The drawing under review shows one solid part. Ordinate dimensions are in mm from its lowest x, y, z. A direction names the side the tool comes from. Give positions to 0.01 mm unless a question says otherwise; leave off trailing zeros. Order: outer loops, then holes, each group sorted by start corner. A loop starts at its lowest first (then second) coordinate and runs counter-clockwise, first axis right, second up. Notation, with made-up numbers: (-14.75, -12) - (37.25, -12) arc R23 ccw to (37.25, 12) - close; hole circle Ø2 at (2.5, -20.5). An arc over 180 degrees is marked (long way). Use CSV: the item, a comma, the result in double quotes.
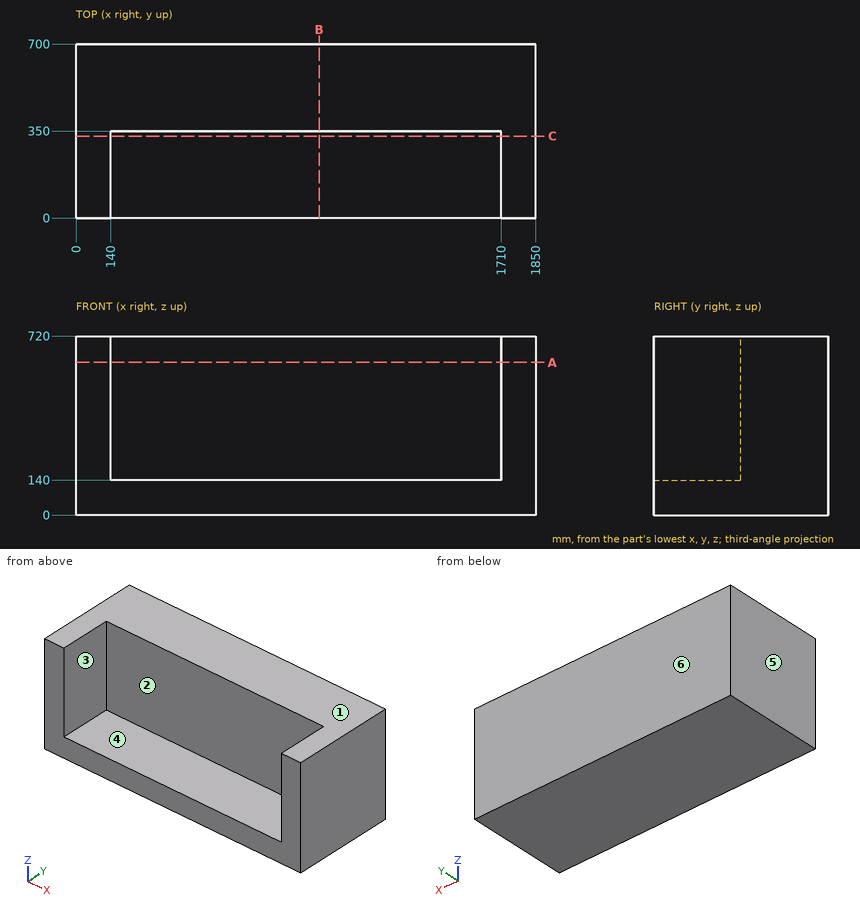
Item 1: Take a section at B-B, the plane x = 977.5. Give the boundary of the cut face in (y, z), and give its area (3 significant figures).
Results list:
outline,"(0, 0) - (700, 0) - (700, 720) - (350, 720) - (350, 140) - (0, 140) - close"
area,"301,000 mm2"
Item 2: Clearance check with a flat-ended pin moving along its axis: pin 1 (10 mm diameter, centred on x = 465, y = 264.5, fed in from +Z). State where the tip first meets the part, or that it passes through.
Results list:
pin 1,"stops at z = 140"
Item 3: Take a section at C-C, the plane y = 329.5. Give the boundary of the cut face in (x, z), and give its area (3 significant figures).
Results list:
outline,"(0, 0) - (1850, 0) - (1850, 720) - (1710, 720) - (1710, 140) - (140, 140) - (140, 720) - (0, 720) - close"
area,"421,000 mm2"
Item 4: Take a section at A-A, the plane z = 614.5. Give the boundary of the cut face in (x, y).
Results list:
outline,"(0, 0) - (140, 0) - (140, 350) - (1710, 350) - (1710, 0) - (1850, 0) - (1850, 700) - (0, 700) - close"
Item 5: Tool access review of the marked faces 1 and 2: name each direction out of +Z, -Z, +X, -X, +Y, -Y from which nothing blocks a thin tool from reaching the whole face with its end or side.
Results list:
face 1,"+Z, +X, -X, +Y, -Y"
face 2,"+Z, -Y"
Item 6: Mouldability with a two-part tool opening along X and no side actions: class the marked faces 3, 4, 5 and 6 as pulls with the +X half, pulls with the -X half, needs draft (parallel to the pull), parting line crosses it, or undercut.
Results list:
face 3,"undercut"
face 4,"undercut"
face 5,"pulls with the -X half"
face 6,"needs draft"
Item 7: Wall thickness on L1, parallel to X at y = 253.5, z = 201; L2, parallel to Y at x = 1503, z = 243; L3, parallel to Z at x = 1359, y = 119: over which ranges is each line inside the solid? List them lowest first.
Results list:
L1,"x = 0 to 140, 1710 to 1850"
L2,"y = 350 to 700"
L3,"z = 0 to 140"
